Autodesk Inventor part; units mm, degrees
ref_plane "YZ Plane" through (0, 0, 0) normal (1, 0, 0) x (0, 1, 0)
ref_plane "XZ Plane" through (0, 0, 0) normal (0, 1, 0) x (-1, 0, 0)
ref_plane "XY Plane" through (0, 0, 0) normal (0, 0, 1) x (1, 0, 0)
sketch "Sketch1" plane through (0, 0, 0) normal (0, 0, 1) x (1, 0, 0)
  circle A0 centre (0, 0) radius 40
  circle A1 centre (0, 0) radius 15
  circle A2 centre (0, 0) radius 35 construction
  line L0 (0, 0) -> (0, 35) construction
  line L1 (0, 0) -> (13.3939, 32.3358) construction
  dimension "d0" = 80
  dimension "d1" = 30
  dimension "d2" = 70
  dimension "d3" = 22.5
extrude "Extrusion1" add sketch "Sketch1" along normal blind 5
hole "Hole1" at (0, 35, 0) direction (0, 0, 1) diameter 4.5 depth 11.8
pattern_circular "Circular Pattern1" count 8 over 360 about axis through (0, 0, -10) along (0, 0, 1) of "Hole1"
chamfer "Chamfer1" distance 0.5 angle 45 2 edges at (-40, 0, 5) (-15, 0, 5)
properties part number "PWTR-0070" material "Stainless Steel"
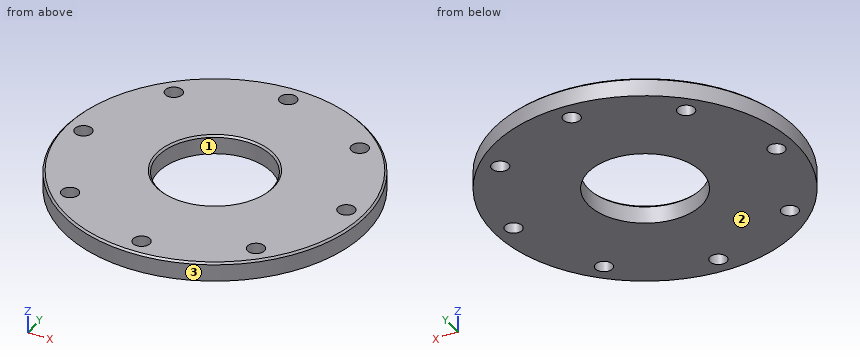
Geometry: final body of the model. Coordinates: model frame, mm. Face numbers are marked on the shaded views. Give positions to 0.01 mm unless a question says otherwise; leave off trailing zeros. Write each loop counter-clockwise with the first axis right and the second up, starting at its lowest first coordinate (ties: lowest second). Pieces come first, ordered by that corner, then holes. Notation, with made-up numbers: (8, 89) -> (61, 89) arc R19 cw to (61, 93) -> close; hole circle Ø10 at (53, 21). An arc over 180 degrees is marked (long way). Answer as a JSON object with one key per item and string values.
1. Mould query, pull axis X, two halves, no side actions, for the marked faces 1, 2 and 3. Classes: pulls with the +X half, pulls with the -X half, needs draft (parallel to the pull), parting line crosses it, or undercut.
Ans:
{"face 1": "undercut", "face 2": "needs draft", "face 3": "parting line crosses it"}
2. Ray query, probe 1 along X at (y, z) = (1, 4.75); probe 2 along Y at (x, z) = (-26.5, 4.1); probe 3 along X at (y, z) = (-1.5, 3.1). Return the intervals inside material, ascending. Write a range as from..to.
Ans:
{"probe 1": "x = -39.74..-37.02, -32.98..-15.22, 15.22..32.98, 37.02..39.74", "probe 2": "y = -29.96..-26.16, -23.34..23.34, 26.16..29.96", "probe 3": "x = -39.97..-36.68, -33.32..-14.92, 14.92..33.32, 36.68..39.97"}
3. Cut plane C-C on z = 2.5. Count the separate pieces of the cut face and the enclosed holes in it, and give its area (3 significant figures).
Ans:
{"separate pieces": "1", "enclosed holes": "9", "area": "4,190 mm^2"}
4. Contact query for flat-ended pins moving along their axis: pin 1 (4 mm diameter, centred on x = -24.75, y = 24.75, fed in from +Z); pin 2 (3 mm diameter, centred on y = -23.5, z = 3, fed in from -X); pin 3 (1.5 mm diameter, centred on x = 15.5, z = 3, fed in from +Y). Output: stop coordinate, or through.
Ans:
{"pin 1": "passes through", "pin 2": "stops at x = -33.41", "pin 3": "stops at y = 37.18"}
5. Cut plane A-A on y = 0. Output: boundary loops of the cut face in (x, z), and give its area (4 significant figures).
Ans:
{"outline": "(-40, 0) -> (-37.25, 0) -> (-37.25, 5) -> (-39.5, 5) -> (-40, 4.5) -> close; (-32.75, 0) -> (-15, 0) -> (-15, 4.5) -> (-15.5, 5) -> (-32.75, 5) -> close; (15, 0) -> (32.75, 0) -> (32.75, 5) -> (15.5, 5) -> (15, 4.5) -> close; (37.25, 0) -> (40, 0) -> (40, 4.5) -> (39.5, 5) -> (37.25, 5) -> close", "area": "204.5 mm^2"}
